```python
from build123d import *

# Parameters (mm, degrees)
F0_W     = 101.6
F0_H     = 63.5
F1_DEPTH = 63.5
F2_W     = 76.2
F2_H     = 12.7
F3_DEPTH = 63.5
F4_W     = 25.4
F4_H     = 25.4
F5_DEPTH = 63.5
F6_W     = 25.4
F6_H     = 25.4
F7_DEPTH = 63.5


with BuildPart() as f1:
    # F0 (on Front) → F1 (new body)
    with BuildSketch(Plane.XZ):
        with Locations((50.8, -31.75)):
            Rectangle(F0_W, F0_H)
    extrude(amount=F1_DEPTH)

    # F2 (on face) → F3 (cut)
    with BuildSketch(Plane.XZ.offset(63.5)):
        with Locations((50.8, -57.15)):
            Rectangle(F2_W, F2_H)
    extrude(amount=-F3_DEPTH, mode=Mode.SUBTRACT)

    # F4 (on face) → F5 (cut)
    with BuildSketch(Plane.XZ.offset(63.5)):
        with Locations((88.9, -12.7)):
            Rectangle(F4_W, F4_H)
    extrude(amount=-F5_DEPTH, mode=Mode.SUBTRACT)

    # F6 (on face) → F7 (cut)
    with BuildSketch(Plane.XZ.offset(63.5)):
        with Locations((12.7, -12.7)):
            Rectangle(F6_W, F6_H)
    extrude(amount=-F7_DEPTH, mode=Mode.SUBTRACT)


solid = f1.part
```
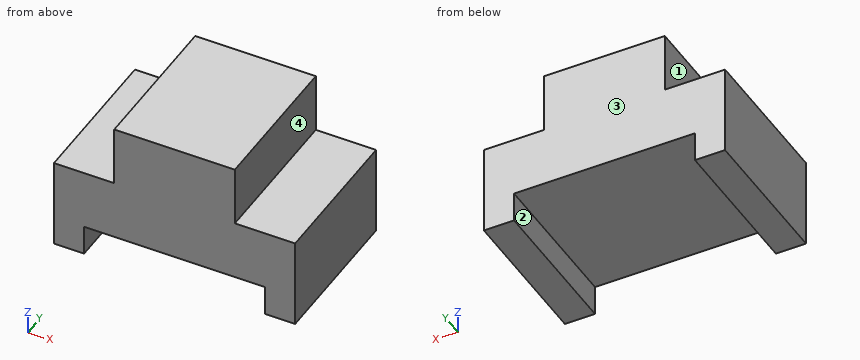
Source: CAD feature listing. Evaluate the final solid. Frame: model axes, mm. Face numbers are marked on the shaded views. A direction names the side the tool comes from. Give positions to 0.01 mm unless a question says otherwise; leave off trailing zeros. Loops run counter-clockwise (first coordinate to the right, second up) from the corner with the lowest first, then second, coordinate; pieces in that order, holes last. Notation, with made-up numbers: (13.5, 29) -> (65.5, 29) arc R7 ccw to (65.5, 40) -> close; hole circle Ø6 at (85.5, -34). An arc over 180 degrees is marked (long way). Put each result on its own line as item: value. Start each with the question number.
1) Contact query for flat-ended pins moving along their axis: P1, Ø7.5, axis at y = -33, z = -14, coming from the +X side; P2, Ø12.5, axis at x = 6.5, y = -21.5, coming from the +Z side; P3, Ø12.5, axis at y = -30.5, z = -13.5, coming from the -X side. Output: stop coordinate, or through.
2) Cut plane B-B (y = -11). Return loops of the section in (x, z).
3) Cut plane D-D (z = -15.5). Return loops of the section in (x, y).
4) Cut plane C-C (x = 94). Return loops of the section in (y, z).
5) Reachability of the marked faces 1, 2, 3 and 4 from +Z, -Z, +X, -X, +Y, -Y: full face, straight path, thin tool, end or side. Return the list, or none.
6) Material intervals for probe 1 along Z at (x, y) = (71.5, -50.5); probe 2 along Z at (x, y) = (16.5, -14.5); probe 3 along X at (y, z) = (-32, -58.5), sorted ascending.
7) Cut plane A-A (z = -56). Return loops of the section in (x, y), then the cut area to 3 significant figures.
Results are:
1. P1: stops at x = 76.2
1. P2: stops at z = -25.4
1. P3: stops at x = 25.4
2. outline: (0, -63.5) -> (12.7, -63.5) -> (12.7, -50.8) -> (88.9, -50.8) -> (88.9, -63.5) -> (101.6, -63.5) -> (101.6, -25.4) -> (76.2, -25.4) -> (76.2, 0) -> (25.4, 0) -> (25.4, -25.4) -> (0, -25.4) -> close
3. outline: (25.4, -63.5) -> (76.2, -63.5) -> (76.2, 0) -> (25.4, 0) -> close
4. outline: (-63.5, -63.5) -> (0, -63.5) -> (0, -25.4) -> (-63.5, -25.4) -> close
5. face 1: +Z, -X, +Y, -Y
5. face 2: -Z, +Y, -Y
5. face 3: +Z, -Z, +X, -X, +Y
5. face 4: +Z, +X, +Y, -Y
6. probe 1: z = -50.8 to 0
6. probe 2: z = -50.8 to -25.4
6. probe 3: x = 0 to 12.7, 88.9 to 101.6
7. outline: (0, -63.5) -> (12.7, -63.5) -> (12.7, 0) -> (0, 0) -> close; (88.9, -63.5) -> (101.6, -63.5) -> (101.6, 0) -> (88.9, 0) -> close
7. area: 1,610 mm2
